Geometry check sheet. Reference: the model listing, model coordinates, mm. Give positions to 0.01 mm unless a question says otherwise; leave off trailing zeros. Write each loop counter-clockwise with the first axis right and the second up, starting at its lowest first coordinate (ties: lowest second). Pieces come first, ordered by that corner, then holes. Notation, with made-up numbers: (31, -25.75) - (68, -25.75) arc R19 cw to (68, 4.25) - close; hole circle Ø4 at (-21.75, -26.75). An arc over 180 degrees is marked (long way). Write item = value, one per line. Start each with the question number.
(1) Draft check along Z on faces 1 (the flat face through (6.38, -3.45, -12.65)), 2 (the flat face through (-10.384, -3.35, 21.552)), 3 (the flat face through (-5.78, -3.45, 55.43)). Enter one of: pulls with the +Z half, pulls with the -Z half, needs draft (parallel to the pull), parting line crosses it, or undercut.
(2) Section check C-C, the plane x = -4.75. Enter the section's corners in (y, z), plus the area to 3 significant figures.
(3) Section check B-B, the plane y = -2. Enter the section's corners in (x, z), plus the area to 3 significant figures.
(4) Depth check by flat-ended pin: pin 1 Ø1.5 at (y, z) = (-3, 22) entering from +X; pin 2 Ø2 at (x, y) = (-8.5, -4) entering from -Z. Enter the tip coordinate at first touch or a pass-through.
(5) Thickness scan on L1, parallel to Z at x = 9, y = -3; L2, parallel to Z at x = 0.5, y = -5.75; L3, parallel to X at y = -6.5, z = -1. Record the ranges inside material, lowest first.
(6) Section check D-D, the plane y = -5.25. Enter the section's corners in (x, z).
(7) Section check A-A, the plane z = 2. Enter the section's corners in (x, y), plus the area to 3 significant figures.
```python
from build123d import *

# Parameters (mm, degrees)
BOSS_EXTRUDE1_START = -22
BOSS_EXTRUDE1_DEPTH = 80
SKETCH3_OUTSIDE_W   = 42.192
SKETCH3_OUTSIDE_H   = 98.732
CUT_EXTRUDE1_DEPTH  = 60.586928072


with BuildPart() as part:
    # Sketch2 → Boss-Extrude1 (new body)
    with BuildSketch(Plane.XY.offset(BOSS_EXTRUDE1_START)):
        Polygon((9, 0), (11.730387764, -6.607891004), (11.336920491, -7), (-11.336920491, -7), (-11.730387764, -6.607891004), (-9, 0), align=None)
    extrude(amount=BOSS_EXTRUDE1_DEPTH)

    # Sketch3 outside → Cut-Extrude1 (cut, through all)
    with BuildSketch(Plane(origin=(0, 0, 0), x_dir=(1, 0, 0), z_dir=(0, 1, 0))):
        with Locations((0, -18)):
            Rectangle(SKETCH3_OUTSIDE_W, SKETCH3_OUTSIDE_H)
        Polygon((-11.730387764, 7.23737522), (-3.070013885, 16), (-1.5, 22), (1.5, 22), (3.070013885, 16), (11.730387764, 7.23737522), (11.730387764, -52.786494327), (0, -58), (-11.730387764, -52.786494327), align=None, mode=Mode.SUBTRACT)
    extrude(amount=-CUT_EXTRUDE1_DEPTH, mode=Mode.SUBTRACT)


solid = part.part
```
Model answer:
q1.face_1 = pulls with the -Z half
q1.face_2 = needs draft
q1.face_3 = pulls with the +Z half
q2.outline = (-7, -14.3) - (0, -14.3) - (0, 55.89) - (-7, 55.89) - close
q2.area = 491 mm²
q3.outline = (-9.83, -9.16) - (-3.07, -16) - (-1.5, -22) - (1.5, -22) - (3.07, -16) - (9.83, -9.16) - (9.83, 53.63) - (0, 58) - (-9.83, 53.63) - close
q3.area = 1,390 mm²
q4.pin_1 = 10.55
q4.pin_2 = -11.52
q5.L1 = -10 to 54
q5.L2 = -22 to 57.78
q5.L3 = -11.69 to 11.69
q6.outline = (-11.17, -7.81) - (-3.07, -16) - (-1.5, -22) - (1.5, -22) - (3.07, -16) - (11.17, -7.81) - (11.17, 53.04) - (0, 58) - (-11.17, 53.04) - close
q7.outline = (-11.73, -6.61) - (-11.34, -7) - (11.34, -7) - (11.73, -6.61) - (9, 0) - (-9, 0) - close
q7.area = 146 mm²
